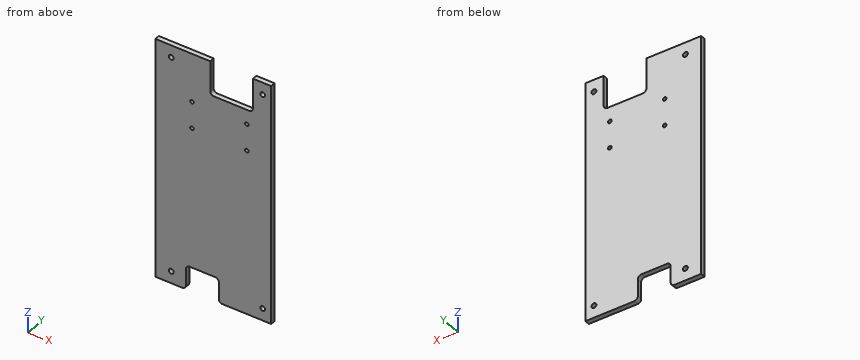
```python
from build123d import *

# Parameters (mm, degrees)
SKETCH_1_W          = 95
SKETCH_1_H          = 198
EXTRUDE_1_DEPTH     = 4
SKETCH_2_W          = 35
SKETCH_2_H          = 28
CUT_EXTRUDE_1_DEPTH = 4
SKETCH_3_R          = 2
CUT_EXTRUDE_2_DEPTH = 110.878341815
SKETCH_4_R          = 2
CUT_EXTRUDE_3_DEPTH = 110.878341815
SKETCH_5_W          = 27
SKETCH_5_H          = 20
CUT_EXTRUDE_4_DEPTH = 110.878341815
SKETCH_6_R          = 1.5
CUT_EXTRUDE_5_DEPTH = 20
FILLET_1_R          = 3
FILLET_2_R          = 3


with BuildPart() as part:
    # 草图1 → 凸台-拉伸1 (new body)
    with BuildSketch(Plane(origin=(0, 0, 0), x_dir=(1, 0, 0), z_dir=(0, 1, 0))):
        Rectangle(SKETCH_1_W, SKETCH_1_H)
    extrude(amount=EXTRUDE_1_DEPTH)

    # 草图2 → 切除-拉伸1 (cut)
    with BuildSketch(Plane(origin=(0, 4, 0), x_dir=(1, 0, 0), z_dir=(0, 1, 0))):
        with Locations((15, -85)):
            Rectangle(SKETCH_2_W, SKETCH_2_H)
    extrude(amount=-CUT_EXTRUDE_1_DEPTH, mode=Mode.SUBTRACT)

    # 草图3 → 切除-拉伸2 (cut, through all)
    with BuildSketch(Plane(origin=(0, 4, 0), x_dir=(1, 0, 0), z_dir=(0, 1, 0))):
        with Locations(Location((40.5, -89, 0), (0, 0, 270))):
            Circle(SKETCH_3_R)
    extrude(amount=-CUT_EXTRUDE_2_DEPTH, mode=Mode.SUBTRACT)

    # 草图4 → 切除-拉伸3 (cut, through all)
    with BuildSketch(Plane(origin=(0, 4, 0), x_dir=(1, 0, 0), z_dir=(0, 1, 0))):
        with Locations(Location((40.5, 89, 0), (0, 0, 270))):
            Circle(SKETCH_4_R)
        with Locations(Location((-34.5, 89, 0), (0, 0, 270))):
            Circle(SKETCH_4_R)
        with Locations(Location((-34.5, -89, 0), (0, 0, 270))):
            Circle(SKETCH_4_R)
    extrude(amount=-CUT_EXTRUDE_3_DEPTH, mode=Mode.SUBTRACT)

    # 草图5 → 切除-拉伸4 (cut, through all)
    with BuildSketch(Plane(origin=(0, 4, 0), x_dir=(1, 0, 0), z_dir=(0, 1, 0))):
        with Locations((-9, 89)):
            Rectangle(SKETCH_5_W, SKETCH_5_H)
    extrude(amount=-CUT_EXTRUDE_4_DEPTH, mode=Mode.SUBTRACT)

    # 草图6 → 切除-拉伸5 (cut)
    with BuildSketch(Plane(origin=(0, 4, 0), x_dir=(1, 0, 0), z_dir=(0, 1, 0))):
        with Locations(Location((-17.5, -59, 0), (0, 0, 270))):
            Circle(SKETCH_6_R)
        with Locations(Location((27.5, -59, 0), (0, 0, 270))):
            Circle(SKETCH_6_R)
        with Locations(Location((27.5, -37, 0), (0, 0, 270))):
            Circle(SKETCH_6_R)
        with Locations(Location((-17.5, -37, 0), (0, 0, 270))):
            Circle(SKETCH_6_R)
    extrude(amount=-CUT_EXTRUDE_5_DEPTH, mode=Mode.SUBTRACT)

    # 圆角1
    fillet_1_edges = [part.edges().sort_by_distance(p)[0] for p in [
        (-2.5, 2, 71),
        (32.5, 2, 71),
    ]]
    fillet(fillet_1_edges, radius=FILLET_1_R)

    # 圆角2
    fillet_2_edges = [part.edges().sort_by_distance(p)[0] for p in [
        (-22.5, 2, -99),
        (4.5, 2, -99),
        (4.5, 2, -79),
        (-22.5, 2, -79),
    ]]
    fillet(fillet_2_edges, radius=FILLET_2_R)


solid = part.part
```
Could you check a few things on this model? Use its own coordinates, in mm. Coordinates: 2 decimals unless noted, no trailing zeros. Write each loop counter-clockwise with the first axis right and the second up, starting at its lowest first coordinate (ties: lowest second). Pieces come first, ordered by that corner, then holes. Notation, with made-up numbers: (78, 74.5) -> (133, 74.5) arc R19 ccw to (133, 78.5) -> close; hole circle Ø3 at (17, -12). An arc over 180 degrees is marked (long way). Write item = value, one per line. Start each with the question number.
(1) I want a section at C-C (z = 82). Please give me the cut outline in (x, y).
(2) Will this pin go through, and if not, where does the flat tip stop? pin 1 (1.2 mm diameter, centred on x = -4.5, y = 2, fed in from -Z).
(3) I need wall thicknesses on line 1 (X direction, y = 1.6, z = -89); line 2 (X direction, y = 1.85, z = 89); line 3 (X direction, y = 2.3, z = 59). Which ranges of each line are inside material? Lowest first, please. Write a range as [from, to].
(4) I want a section at A-A (z = -89). Please give me the cut outline in (x, y), plus the area to 3 significant figures.
(5) I want a section at D-D (y = 1.5). Give the number of separate pieces and of enclosed holes in the cut face, plus the area to 3 significant figures.
(6) I want a section at B-B (x = 40.5). Please give me the cut outline in (y, z), plus the area to 3 significant figures.
Result set:
q1.outline = (-47.5, 0) -> (-2.5, 0) -> (-2.5, 4) -> (-47.5, 4) -> close; (32.5, 0) -> (47.5, 0) -> (47.5, 4) -> (32.5, 4) -> close
q2.pin_1 = -79
q3.line_1 = [-47.5, -36.5], [-32.5, -22.5], [4.5, 38.5], [42.5, 47.5]
q3.line_2 = [-47.5, -36.5], [-32.5, -2.5], [32.5, 38.5], [42.5, 47.5]
q3.line_3 = [-47.5, -19], [-16, 26], [29, 47.5]
q4.outline = (-47.5, 0) -> (-36.5, 0) -> (-36.5, 4) -> (-47.5, 4) -> close; (-32.5, 0) -> (-22.5, 0) -> (-22.5, 4) -> (-32.5, 4) -> close; (4.5, 0) -> (38.5, 0) -> (38.5, 4) -> (4.5, 4) -> close; (42.5, 0) -> (47.5, 0) -> (47.5, 4) -> (42.5, 4) -> close
q4.area = 240 mm2
q5.separate_pieces = 1
q5.enclosed_holes = 8
q5.area = 17,200 mm2
q6.outline = (0, -99) -> (4, -99) -> (4, -91) -> (0, -91) -> close; (0, -87) -> (4, -87) -> (4, 87) -> (0, 87) -> close; (0, 91) -> (4, 91) -> (4, 99) -> (0, 99) -> close
q6.area = 760 mm2
